Geometry check sheet. Reference: the model listing, model coordinates, mm. A direction names the side the tool comes from. Give positions to 0.01 mm unless a question says otherwise; leave off trailing zeros. Order: outer loops, then holes, each group sorted by start corner. A loop starts at its lowest first (then second) coordinate and runs counter-clockwise, first axis right, second up. Notation, with made-up numbers: M -37.75,43 L -9.75,43 A29 ccw -9.75,75 Z; hole C -22,88 d11. An arc over 180 degrees is marked long. Answer as CSV lines item,"result".
from build123d import *

# Parameters (mm, degrees)
F0_R     = 22
F0_R_2   = 20
F1_DEPTH = 33
F2_R     = 22
F2_R_2   = 2.5
F3_DEPTH = 2
F5_DEPTH = 2
F6_R     = 4
F6_R_2   = 2.5
F7_DEPTH = 1.5


with BuildPart() as f1:
    # F0 (on Top) → F1 (new body)
    with BuildSketch(Plane.XY):
        Circle(F0_R)
        Circle(F0_R_2, mode=Mode.SUBTRACT)
    extrude(amount=F1_DEPTH)

    # F2 (on Top) → F3 (join)
    with BuildSketch(Plane.XY):
        Circle(F2_R)
        Circle(F2_R_2, mode=Mode.SUBTRACT)
    extrude(amount=F3_DEPTH)

    # F4 (on face) → F5 (cut)
    with BuildSketch(Plane.XY.offset(33)):
        with BuildLine():
            Line((-3.106676, 21.803428), (-2.5, 19.843135))
            ThreePointArc((-2.5, 19.843135), (-1.252458, 19.960745), (0, 20))
            ThreePointArc((0, 20), (1.252458, 19.960745), (2.5, 19.843135))
            Line((2.5, 19.843135), (3.106676, 21.803428))
            ThreePointArc((3.106676, 21.803428), (0, 22.023645), (-3.106676, 21.803428))
        make_face()
        with BuildLine():
            Line((-21.803428, -3.106676), (-19.843135, -2.5))
            ThreePointArc((-19.843135, -2.5), (-19.960745, -1.252458), (-20, 0))
            ThreePointArc((-20, 0), (-19.960745, 1.252458), (-19.843135, 2.5))
            Line((-19.843135, 2.5), (-21.803428, 3.106676))
            ThreePointArc((-21.803428, 3.106676), (-22.023645, 0), (-21.803428, -3.106676))
        make_face()
        with BuildLine():
            Line((3.106676, -21.803428), (2.5, -19.843135))
            ThreePointArc((2.5, -19.843135), (1.252458, -19.960745), (0, -20))
            ThreePointArc((0, -20), (-1.252458, -19.960745), (-2.5, -19.843135))
            Line((-2.5, -19.843135), (-3.106676, -21.803428))
            ThreePointArc((-3.106676, -21.803428), (0, -22.023645), (3.106676, -21.803428))
        make_face()
        with BuildLine():
            Line((21.803428, 3.106676), (19.843135, 2.5))
            ThreePointArc((19.843135, 2.5), (19.960745, 1.252458), (20, 0))
            ThreePointArc((20, 0), (19.960745, -1.252458), (19.843135, -2.5))
            Line((19.843135, -2.5), (21.803428, -3.106676))
            ThreePointArc((21.803428, -3.106676), (22.023645, 0), (21.803428, 3.106676))
        make_face()
    extrude(amount=-F5_DEPTH, mode=Mode.SUBTRACT)

    # F6 (on face) → F7 (join)
    with BuildSketch(Plane.XY.offset(2)):
        Circle(F6_R)
        Circle(F6_R_2, mode=Mode.SUBTRACT)
    extrude(amount=F7_DEPTH)


solid = f1.part
(1) Section check A-A on x = 0. Enter the section's corners in (y, z), then the cut area to 4 significant figures.
The answers:
outline,"M -22,0 L -2.5,0 L -2.5,3.5 L -4,3.5 L -4,2 L -20,2 L -20,31 L -22,31 Z; M 2.5,0 L 22,0 L 22,31 L 20,31 L 20,2 L 4,2 L 4,3.5 L 2.5,3.5 Z"
area,"198.5 mm2"
(2) Section check C-C on y = -11. Enter the section's corners in (x, z), then the cut area to 3 significant figures.
The answers:
outline,"M -19.05,0 L 19.05,0 L 19.05,33 L 16.7,33 L 16.7,2 L -16.7,2 L -16.7,33 L -19.05,33 Z"
area,"222 mm2"
(3) Tool access check on faces 1 (the face through (2.804, -20.825, 32.014)), 2 (the face through (2.796, 20.798, 32.014)), 3 (the face through (-20.798, 2.796, 32.014)), 4 (the face through (2, 2, 3.5)), 5 (the face through (21, 0, 31)). Record the directions out of +Z, -Z, +X, -X, +Y, -Y that give a thin tool (end or side, any length) a straight path to the whole face; none if there is none.
The answers:
face 1,"+Z, -Y"
face 2,"+Z, +Y"
face 3,"+Z, -X"
face 4,"+Z"
face 5,"+Z, +X"
(4) Material ranges on line 1 (X direction, y = 0, z = 11); line 2 (Y direction, x = 0, z = 1.1), recorded low to high.
The answers:
line 1,"x = -22 to -20, 20 to 22"
line 2,"y = -22 to -2.5, 2.5 to 22"
(5) Draft check along Y on faces 6 (the face through (-2.804, 20.825, 32.014)), 7 (the face through (-14.3, 14.3, 33)), 8 (the face through (4.2, 0.3, 2)). Enter one of: +Y half, -Y half, draft (parallel to the pull), parting line (faces both ways), or undercut.
The answers:
face 6,"+Y half"
face 7,"draft"
face 8,"undercut"
(6) Gauge pin test, flat ends, axial feed: P1, Ø0.6, axis at x = 21, y = -1.5, coming from the +Z side; P2, Ø12, axis at x = -1.5, y = 3, coming from the +Z side; P3, Ø12, axis at x = -9.5, y = -5, coming from the +Z side. Record the tip position at first contact, or that the pin passes through.
The answers:
P1,"stops at z = 31"
P2,"stops at z = 3.5"
P3,"stops at z = 2"
(7) Section check D-D on z = 9.5. Enter the section's corners in (x, y).
The answers:
outline,"C 0,0 d44; hole C 0,0 d40"
